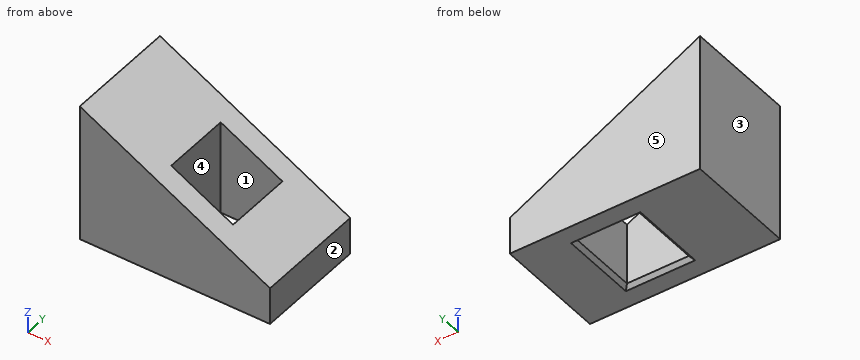
```python
from build123d import *

# Parameters (mm, degrees)
F0_W     = 25.4
F0_H     = 15.0114
F0_W_2   = 8.25
F0_H_2   = 9.25
F1_DEPTH = 18.5
F3_DEPTH = 25.4
F4_SIZE  = 0.508


with BuildPart() as f1:
    # F0 (on Top) → F1 (new body)
    with BuildSketch(Plane.XY):
        Rectangle(F0_W, F0_H)
        with Locations((1.585, 0)):
            Rectangle(F0_W_2, F0_H_2, mode=Mode.SUBTRACT)
    extrude(amount=F1_DEPTH)

    # F2 (on face) → F3 (cut)
    with BuildSketch(Plane.XZ.offset(7.5057)):
        Polygon((12.7, 18.5), (-12.7, 18.5), (12.7, 4.97428), align=None)
    extrude(amount=-F3_DEPTH, mode=Mode.SUBTRACT)

    # F4
    f4_edges = [f1.edges().sort_by_distance(p)[0] for p in [
        (-2.54, 0, 0),
        (1.585, 4.625, 0),
        (5.71, 0, 0),
        (1.585, -4.625, 0),
    ]]
    chamfer(f4_edges, length=F4_SIZE)


solid = f1.part
```
Verification items for the finished model (mm, model axes). Face numbers are marked on the shaded views. A direction names the side the tool comes from. Give positions to 0.01 mm unless a question says otherwise; leave off trailing zeros. Order: outer loops, then holes, each group sorted by start corner. A loop starts at its lowest first (then second) coordinate and runs counter-clockwise, first axis right, second up. Notation, with made-up numbers: M 53,40.5 L 112,40.5 A17 cw 112,46.5 Z; hole C -30.5,55 d4. An arc over 180 degrees is marked long. Answer in a Markdown table with one row per item. Add a question column.
Item 1: Section check A-A, the plane y = -4.25. Enter the section's corners in (x, z), and give its area (3 significant figures).
Item 2: Mould release check, pull along X, two halves, no side actions. Record for the marked faces 3, 4 and 5: released by +X, released by -X, zero draft, split by the parting line, or undercut.
Item 3: Tool access check on the marked faces 1 and 2. Record the directions out of +Z, -Z, +X, -X, +Y, -Y that give a thin tool (end or side, any length) a straight path to the whole face; none if there is none.
Item 4: Section check D-D, the plane z = 7. Enter the section's corners in (x, y) (3 decimals), and give its area (3 significant figures).
Item 5: Gauge pin test, flat ends, axial feed: pin 1 (3 mm diameter, centred on x = -1, y = -0.5, fed in from -Z); pin 2 (1 mm diameter, centred on y = 4, z = 5, fed in from +X); pin 3 (5 mm diameter, centred on x = 4.5, y = 5.5, fed in from +Z). Record the tip position at first contact, or that the pin passes through.
Item 6: Section check C-C, the plane x = 0. Enter the section's corners in (y, z) (3 decimals), and give its area (3 significant figures).
Item 7: Section check B-B, the plane z = 1.5. Enter the section's corners in (x, y) (3 decimals).
Item 8: Scan lines: probe 1 along Y at (x, z) = (5, 7.25) (3 decimals); probe 2 along X at (y, z) = (3.25, 3.5); probe 3 along X at (y, z) = (2.75, 11). Record each from-to range of solid material in increasing order. Write a range as from..to.
Filled sheet:
| question | item | result |
|---|---|---|
| 1 | outline | M -12.7,0 L -3.05,0 L -2.54,0.51 L -2.54,13.09 L -12.7,18.5 Z; M 5.71,0.51 L 6.22,0 L 12.7,0 L 12.7,4.97 L 5.71,8.7 Z |
| 1 | area | 208 mm^2 |
| 2 | face 3 | released by -X |
| 2 | face 4 | undercut |
| 2 | face 5 | zero draft |
| 3 | face 1 | +Z, -Z |
| 3 | face 2 | +Z, -Z, +X, +Y, -Y |
| 4 | outline | M -12.7,-7.506 L 8.896,-7.506 L 8.896,7.506 L -12.7,7.506 Z; hole M -2.54,-4.625 L 5.71,-4.625 L 5.71,4.625 L -2.54,4.625 Z |
| 4 | area | 248 mm^2 |
| 5 | pin 1 | passes through |
| 5 | pin 2 | stops at x = 12.7 |
| 5 | pin 3 | stops at z = 10.67 |
| 6 | outline | M -7.506,0 L -5.133,0 L -4.625,0.508 L -4.625,11.737 L -7.506,11.737 Z; M 4.625,0.508 L 5.133,0 L 7.506,0 L 7.506,11.737 L 4.625,11.737 Z |
| 6 | area | 67.4 mm^2 |
| 7 | outline | M -12.7,-7.506 L 12.7,-7.506 L 12.7,7.506 L -12.7,7.506 Z; hole M -2.54,-4.625 L 5.71,-4.625 L 5.71,4.625 L -2.54,4.625 Z |
| 8 | probe 1 | y = -7.506..-4.625, 4.625..7.506 |
| 8 | probe 2 | x = -12.7..-2.54, 5.71..12.7 |
| 8 | probe 3 | x = -12.7..-2.54 |
